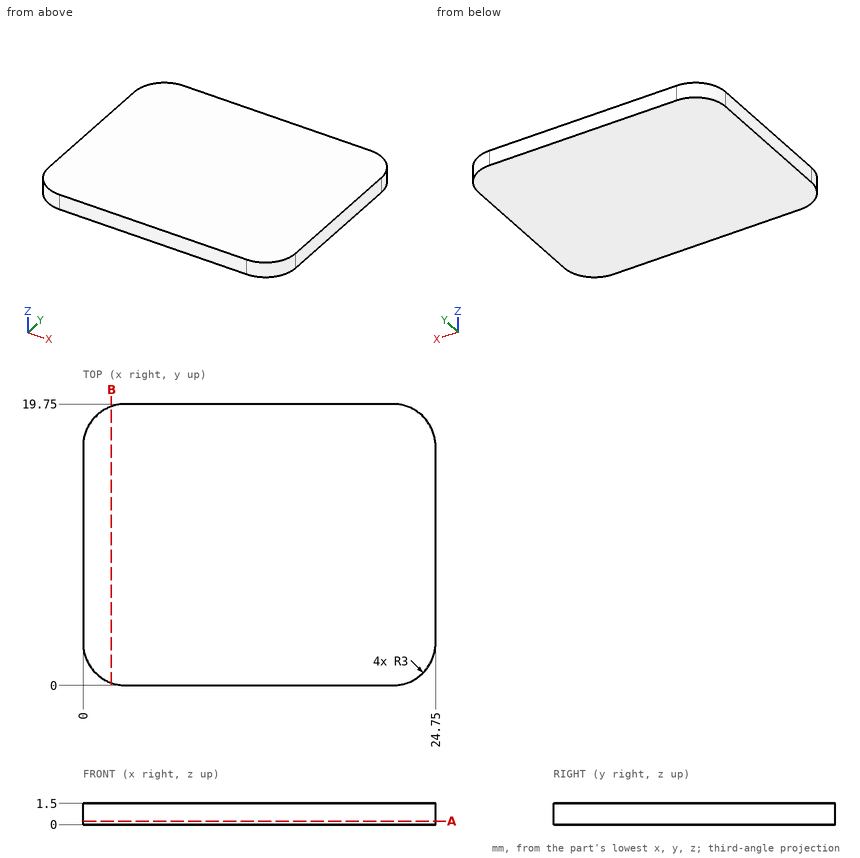
Verification items for this drawing (mm, ordinates from the low corner). Round coordinates to 2 decimals unless told otherwise and drop trailing zeros. Write each loop counter-clockwise with the first axis right and the second up, starting at its lowest first coordinate (ties: lowest second). Pieces come first, ordered by that corner, then holes. Notation, with made-up numbers: (89, 16.25) - (95, 16.25) arc R23 ccw to (95, 50.25) - close; hole circle Ø7 at (13.25, 66.25). An arc over 180 degrees is marked (long way). Answer as a JSON object with one key per item and string values. Group by question number.
Q1. Section check B-B, the plane x = 2. Enter the section's corners in (y, z).
Q2. Thickness scan on line 1 (Y direction, x = 2.25, z = 0.7); line 2 (X direction, y = 17.5, z = 0.35); line 3 (X direction, y = 1.25, z = 0.9). Record the ranges inside material, lowest first.
Q3. Section check A-A, the plane z = 0.25. Enter the section's corners in (x, y), plus the area to 3 significant figures.
Found:
{
 "1": {"outline": "(0.17, 0) - (19.58, 0) - (19.58, 1.5) - (0.17, 1.5) - close"},
 "2": {"line 1": "y = 0.1 to 19.65", "line 2": "x = 0.1 to 24.65", "line 3": "x = 0.56 to 24.19"},
 "3": {"outline": "(0, 3) arc R3 ccw to (3, 0) - (21.75, 0) arc R3 ccw to (24.75, 3) - (24.75, 16.75) arc R3 ccw to (21.75, 19.75) - (3, 19.75) arc R3 ccw to (0, 16.75) - close", "area": "481 mm^2"}
}
